```python
from build123d import *

# Parameters (mm, degrees)
SKETCH_1_W          = 50
SKETCH_1_H          = 50
SKETCH_1_R          = 1.5
EXTRUDE_1_DEPTH     = 3
SKETCH_2_R          = 1
CUT_EXTRUDE_2_DEPTH = 56.982140009
SKETCH_4_R          = 2
CUT_EXTRUDE_4_DEPTH = 50


with BuildPart() as part:
    # 草图1 → 凸台-拉伸1 (new body)
    with BuildSketch(Plane(origin=(0, 0, 0), x_dir=(1, 0, 0), z_dir=(0, 1, 0))):
        Rectangle(SKETCH_1_W, SKETCH_1_H)
        with Locations(Location((0, 10.279455753, 0), (0, 0, 270))):
            Circle(SKETCH_1_R, mode=Mode.SUBTRACT)
        with Locations(Location((8.902269819, -5.139727877, 0), (0, 0, 270))):
            Circle(SKETCH_1_R, mode=Mode.SUBTRACT)
        with Locations(Location((-8.902269819, -5.139727877, 0), (0, 0, 270))):
            Circle(SKETCH_1_R, mode=Mode.SUBTRACT)
    extrude(amount=EXTRUDE_1_DEPTH)

    # 草图2 → 切除-拉伸2 (cut, through all)
    with BuildSketch(Plane(origin=(25, 0, 0), x_dir=(0, 0, -1), z_dir=(1, 0, 0))):
        with Locations((-22, 1.5)):
            Circle(SKETCH_2_R)
    extrude(amount=-CUT_EXTRUDE_2_DEPTH, mode=Mode.SUBTRACT)

    # 草图4 → 切除-拉伸4 (cut)
    with BuildSketch(Plane.XZ):
        with Locations(Location((-7.5, -19.794917773, 0), (0, 0, 270))):
            Circle(SKETCH_4_R)
        with Locations(Location((7.5, -19.794917773, 0), (0, 0, 270))):
            Circle(SKETCH_4_R)
    extrude(amount=-CUT_EXTRUDE_4_DEPTH, mode=Mode.SUBTRACT)


solid = part.part
```
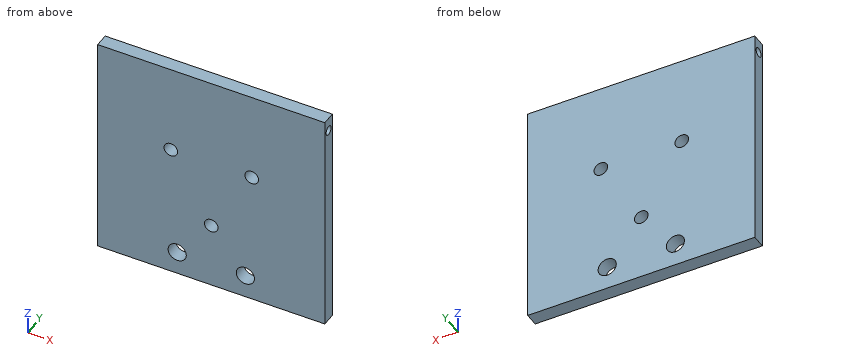
Can you work these out from the model? Positions are in its coordinate system, mm. Round coordinates to 2 decimals unless told otherwise and drop trailing zeros. Loops run counter-clockwise (first coordinate to the right, second up) from the corner with the lowest first, then second, coordinate; pieces in that order, holes last. Notation, with made-up numbers: M 18.25,51 L 65.25,51 A21 cw 65.25,80 Z; hole C 68.25,21.25 d3. An arc over 180 degrees is marked long. Write item = value, one per line. Start each with the question number.
(1) I'm going to push a flat-ended pin straight in: P1, Ø2.5, axis at x = -7.5, z = -19.79, coming from the +Y side. Where does the tip first touch, or does it pass through?
(2) I need wall thicknesses on line 1 along X through (y, z) = (1.85, 5.5); line 2 along Z through (x, y) = (-11.5, 1.4); line 3 along X through (y, z) = (2.4, -11). Which ranges of each line are inside material? Lowest first, please.
(3) Suppose I cut it at A-A on y = 1.5. Write out the boundary of the cut face in (x, z), plus the area to 3 significant figures.
(4) Suppose I cut it at B-B on z = 22. Write out the boundary of the cut face in (x, y), plus the area to 3 significant figures.
(5) Suppose I cut it at C-C on x = 18. Write out the boundary of the cut face in (y, z).
(6) Suppose I cut it at D-D on z = 5. Write out the boundary of the cut face in (x, y), plus the area to 3 significant figures.
Answer block:
q1.P1 = through
q2.line_1 = -25 to -10.36, -7.45 to 7.45, 10.36 to 25
q2.line_2 = -25 to 21.01, 22.99 to 25
q2.line_3 = -25 to -1.32, 1.32 to 25
q3.outline = M -25,-25 L 25,-25 L 25,21 L -25,21 Z; M -25,23 L 25,23 L 25,25 L -25,25 Z; hole C -8.9,5.14 d3; hole C -7.5,-19.79 d4; hole C 0,-10.28 d3; hole C 7.5,-19.79 d4; hole C 8.9,5.14 d3
q3.area = 2,350 mm²
q4.outline = M -25,0 L 25,0 L 25,0.5 L -25,0.5 Z; M -25,2.5 L 25,2.5 L 25,3 L -25,3 Z
q4.area = 50.0 mm²
q5.outline = M 0,-25 L 3,-25 L 3,25 L 0,25 Z; hole C 1.5,22 d2
q6.outline = M -25,0 L -10.4,0 L -10.4,3 L -25,3 Z; M -7.41,0 L 7.41,0 L 7.41,3 L -7.41,3 Z; M 10.4,0 L 25,0 L 25,3 L 10.4,3 Z
q6.area = 132 mm²
